Model file for the job. Use its own axes, mm. Face numbers are marked on the shaded views. A direction names the side the tool comes from. Give positions to 0.01 mm unless a question says otherwise; leave off trailing zeros. Write each loop counter-clockwise with the first axis right and the second up, starting at its lowest first coordinate (ties: lowest second). Pieces come first, ordered by that corner, then holes. Notation, with made-up numbers: (36.5, 41.5) - (89.5, 41.5) arc R12 cw to (89.5, 47.5) - close; hole circle Ø8 at (53, 52.25). An arc over 180 degrees is marked (long way). Use a Markdown table: item, result. Add a question column.
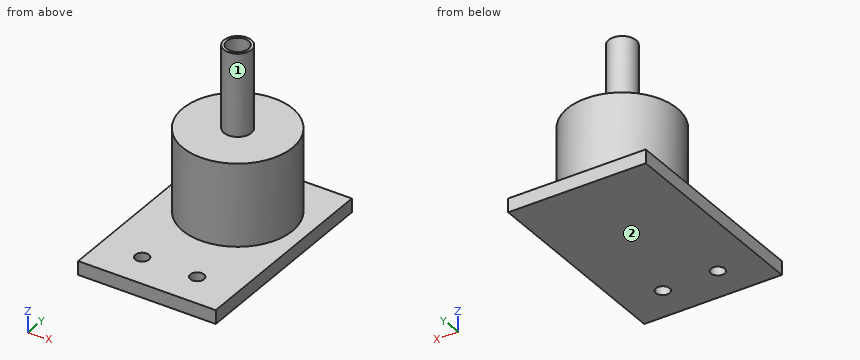
Autodesk Inventor part; units mm, degrees
ref_plane "YZ Plane" through (0, 0, 0) normal (1, 0, 0) x (0, 1, 0)
ref_plane "XZ Plane" through (0, 0, 0) normal (0, 1, 0) x (-1, 0, 0)
ref_plane "XY Plane" through (0, 0, 0) normal (0, 0, 1) x (1, 0, 0)
sketch "Sketch1" plane through (0, 0, 0) normal (0, 0, 1) x (1, 0, 0)
  line L0 (0, 0) -> (50, 0)
  line L1 (50, 0) -> (50, 75)
  line L2 (50, 75) -> (0, 75)
  line L3 (0, 75) -> (0, 0)
  dimension "d0" = 50
  dimension "d1" = 75
extrude "Extrusion1" add sketch "Sketch1" along normal blind 5
sketch "Sketch2" plane through (0, 0, 5) normal (0, 0, 1) x (1, 0, 0)
  line L0 (0, 0) -> (50, 0)
  line L1 (50, 75) -> (0, 75)
  line L2 (0, 0) -> (50, 0)
  line L3 (50, 0) -> (50, 75)
  line L4 (50, 75) -> (0, 75)
  line L5 (0, 75) -> (0, 0)
  circle A0 centre (25, 50) radius 20
  dimension "d4" = 40
  dimension "d5" = 25
extrude "Extrusion2" add sketch "Sketch2" along normal blind 30 contours A0
sketch "Sketch3" plane through (25, 50, 35) normal (0, 0, 1) x (1, 0, 0)
  circle A0 centre (0, 0) radius 4
  circle A1 centre (0, 0) radius 5
  point P0 (-25, -50)
  dimension "d8" = 8
  dimension "d9" = 10
extrude "Extrusion3" add sketch "Sketch3" along normal blind 30
sketch "Sketch4" plane through (0, 0, 5) normal (0, 0, 1) x (1, 0, 0)
  circle A0 centre (35, 12.5) radius 2.5
  circle A1 centre (15, 12.5) radius 2.5
  line L0 (0, 75) -> (0, 0)
  line L1 (50, 0) -> (50, 75)
  line L2 (0, 0) -> (50, 0)
  dimension "d12" = 5
  dimension "d13" = 5
  dimension "d14" = 15
  dimension "d15" = 15
  dimension "d16" = 12.5
  dimension "d17" = 12.5
extrude "Extrusion4" cut sketch "Sketch4" against normal blind 10
thread "Thread1"
thread "Thread2"
properties part number "Pump"
(1) Band-saw the part on B-B (y = 50). Write the cut outline in (x, z), then the cut area to 3 significant figures.
(2) Band-saw the part on C-C (x = 15). Write the cut outline in (y, z).
(3) Band-saw the part on A-A (y = 12.5). Write the cut outline in (x, z).
(4) Probe probe 1 along Y at (x, z) = (25, 53.5); probe 2 along Y at (x, z) = (35, 2.35); probe 3 along X at (y, z) = (12, 3). List the from-to ranges inside material, lowest first. Write a range as [from, to].
(5) Band-saw the part on D-D (z = 60). Write the cut outline in (x, y), then the cut area to 3 significant figures.
(6) Flat gauge pins, fed straight in: pin 1 (10 mm diameter, centred on x = 44, z = 23, fed in from +Y); pin 2 (4 mm diameter, centred on x = 14.5, z = 36.5, fed in from +Y); pin 3 (8 mm diameter, centred on x = 15, y = 12.5, fed in from +Z). Where does each tip first touch, or does it go through?
(7) Which spindle directions (+Z, -Z, +X, -X, +Y, -Y) get a long thin tool onto all of the face, cutting with end or side? Do the marked faces 1 and 2. Say none if no direction does.
Model answer:
| question | item | result |
|---|---|---|
| 1 | outline | (0, 0) - (50, 0) - (50, 5) - (45, 5) - (45, 35) - (30, 35) - (30, 65) - (29, 65) - (29, 35) - (21, 35) - (21, 65) - (20, 65) - (20, 35) - (5, 35) - (5, 5) - (0, 5) - close |
| 1 | area | 1,510 mm^2 |
| 2 | outline | (0, 0) - (10, 0) - (10, 5) - (0, 5) - close; (15, 0) - (75, 0) - (75, 5) - (67.32, 5) - (67.32, 35) - (32.68, 35) - (32.68, 5) - (15, 5) - close |
| 3 | outline | (0, 0) - (12.5, 0) - (12.5, 5) - (0, 5) - close; (17.5, 0) - (32.5, 0) - (32.5, 5) - (17.5, 5) - close; (37.5, 0) - (50, 0) - (50, 5) - (37.5, 5) - close |
| 4 | probe 1 | y = [45, 46], [54, 55] |
| 4 | probe 2 | y = [0, 10], [15, 75] |
| 4 | probe 3 | x = [0, 12.55], [17.45, 32.55], [37.45, 50] |
| 5 | outline | circle Ø10 at (25, 50); hole circle Ø8 at (25, 50) |
| 5 | area | 28.3 mm^2 |
| 6 | pin 1 | stops at y = 64.28 |
| 6 | pin 2 | stops at y = 67.77 |
| 6 | pin 3 | stops at z = 5 |
| 7 | face 1 | +Z |
| 7 | face 2 | -Z, +X, -X, +Y, -Y |
